from build123d import *

# Parameters (mm, degrees)
SKETCH1_W           = 18.734993996
SKETCH1_H           = 15
BOSS_EXTRUDE1_DEPTH = 26
SKETCH2_R           = 6.5
CUT_EXTRUDE1_DEPTH  = 33.32645975
CHAMFER1_SIZE       = 0.5
SKETCH3_R           = 7
BOSS_EXTRUDE2_DEPTH = 4
SKETCH4_R           = 6
BOSS_EXTRUDE3_DEPTH = 11.5
FILLET1_R           = 1.5


with BuildPart() as part:
    # Sketch1 → Boss-Extrude1 (new body)
    with BuildSketch(Plane.XY):
        Rectangle(SKETCH1_W, SKETCH1_H)
        with BuildLine():
            ThreePointArc((-9.367496998, 7.5), (-12, 0), (-9.367496998, -7.5))
            Line((-9.367496998, -7.5), (-9.367496998, 7.5))
        make_face()
        with BuildLine():
            Line((9.367496998, 7.5), (9.367496998, -7.5))
            ThreePointArc((9.367496998, -7.5), (11.322763885, -3.974294656), (12, 0))
            ThreePointArc((12, 0), (11.322763885, 3.974294656), (9.367496998, 7.5))
        make_face()
    extrude(amount=BOSS_EXTRUDE1_DEPTH)

    # Sketch2 → Cut-Extrude1 (cut, through all)
    with BuildSketch(Plane(origin=(0, 7.5, 0), x_dir=(1, 0, 0), z_dir=(0, 1, 0))):
        with Locations(Location((0, -13, 0), (0, 0, 270))):
            Circle(SKETCH2_R)
    extrude(amount=-CUT_EXTRUDE1_DEPTH, mode=Mode.SUBTRACT)

    # Chamfer1
    chamfer1_edges = [part.edges().sort_by_distance(p)[0] for p in [
        (0, -7.5, 6.5),
        (0, 7.5, 6.5),
    ]]
    chamfer(chamfer1_edges, length=CHAMFER1_SIZE)

    # Sketch3 → Boss-Extrude2 (add)
    with BuildSketch(Plane.XY.offset(26)):
        Circle(SKETCH3_R)
    extrude(amount=BOSS_EXTRUDE2_DEPTH)

    # Sketch4 → Boss-Extrude3 (add)
    with BuildSketch(Plane.XY.offset(30)):
        Circle(SKETCH4_R)
    extrude(amount=BOSS_EXTRUDE3_DEPTH)

    # Fillet1
    # the kernel refuses this fillet: 1.5 mm, written as the material it adds along each edge
    with BuildSketch(Plane(origin=(0, 0, 30), x_dir=(1, 0, 0), z_dir=(0, -1, 0))) as fillet1_piece_1:
        with BuildLine():
            CenterArc((7.5, 1.414213562), FILLET1_R, 180, 70.528779366)
            Line((6, 1.414213562), (6, 0))
            Line((6, 0), (7, 0))
        make_face()
    revolve(axis=Axis((0, 0, 30), (0, 0, 1)))
    # the kernel refuses this fillet: 1.5 mm, written as the material it takes off along each edge
    with BuildSketch(Plane(origin=(0, 0, 41.5), x_dir=(1, 0, 0), z_dir=(0, -1, 0))) as fillet1_2_piece_1:
        with BuildLine():
            CenterArc((6 - FILLET1_R, -FILLET1_R), FILLET1_R, 0, 90)
            Line((6 - FILLET1_R, 0), (6, 0))
            Line((6, 0), (6, -FILLET1_R))
        make_face()
    revolve(axis=Axis((0, 0, 41.5), (0, 0, 1)), mode=Mode.SUBTRACT)

    # Mirror1: read off the stored shape, not the designer's step
    # Mirror1 outline → Mirror1 (revolve)
    with BuildSketch(Plane.XZ):
        with BuildLine():
            ThreePointArc((6, -5.414213562), (6.275255129, -4.548188159), (7, -4))
            Line((7, -4), (7, 0))
            Line((7, 0), (0, 0))
            Line((0, 0), (0, -15.5))
            Line((0, -15.5), (4.5, -15.5))
            ThreePointArc((4.5, -15.5), (5.560660172, -15.060660172), (6, -14))
            Line((6, -14), (6, -5.414213562))
        make_face()
    revolve(axis=Axis((0, 0, 0), (0, 0, 1)))


solid = part.part
Design review of the part built by this model. Coordinates are the model's own, in mm. A direction names the side the tool comes from. Give positions to 0.01 mm unless a question says otherwise; leave off trailing zeros. Write each loop counter-clockwise with the first axis right and the second up, starting at its lowest first coordinate (ties: lowest second). Pieces come first, ordered by that corner, then holes. Notation, with made-up numbers: M -15,7 L -8,7 A23 cw -8,17 Z; hole C -38,2.25 d6. An arc over 180 degrees is marked long. Return JSON: item names as keys, results as strings. Group by question number.
Item 1: The part is to be moulded in two halves that separate along X. For faces 1 (the flat face through (0, 0, 41.5)), 2 (the cylindrical face through (-12, 0, 13)), 3 (the cylindrical face through (1.95, 0.1, 19.2)), 4 (the cylindrical face through (-6, 0, -10)), say which applies: pulls with the +X half, pulls with the -X half, needs draft (parallel to the pull), parting line crosses it, or undercut.
Item 2: Wall thickness on line 1 along Z through (x, y) = (-7.25, 2.5); line 2 along Z through (x, y) = (0.75, -3); line 3 along Z through (x, y) = (1.5, 0.75): over which ranges is each line inside the solid? List them lowest first.
Item 3: Clearance check with flat-ended pins moving along their axes: pin 1 Ø12 at (x, z) = (-4.5, 15.5) entering from +Y; pin 2 Ø1 at (y, z) = (-4, 16.5) entering from +X; pin 3 Ø1 at (x, z) = (-3.5, 32) entering from -Y; pin 4 Ø4 at (y, z) = (0, -4.5) entering from -X. State where each tip first meets the part, or that it passes through.
Item 4: Take a section at C-C (z = -9). Give the boundary of the cut face in (x, y).
Item 5: Take a section at A-A (z = 13). Give the boundary of the cut face in (x, y).
Item 6: Take a section at D-D (x = -8.5). Give the boundary of the cut face in (y, z).
Item 7: Tool access review of faces 5 (the flat face through (-3, -7, 26)), 6 (the flat face through (0, 0, -15.5)), 7 (the cylindrical face through (6.466, -2.681, -1.972)): name each direction out of +Z, -Z, +X, -X, +Y, -Y from which nothing blocks a thin tool from reaching the whole face with its end or side.
Return value:
{
 "1": {"face 1": "needs draft", "face 2": "pulls with the -X half", "face 3": "undercut", "face 4": "parting line crosses it"},
 "2": {"line 1": "z = 0 to 26", "line 2": "z = -15.5 to 6.54, 19.46 to 41.5", "line 3": "z = -15.5 to 6.68, 19.32 to 41.5"},
 "3": {"pin 1": "stops at y = 7.5", "pin 2": "stops at x = 11.48", "pin 3": "stops at y = -5.2", "pin 4": "stops at x = -7"},
 "4": {"outline": "C 0,0 d12"},
 "5": {"outline": "M -9.37,-7.5 L -7,-7.5 L -6.5,-7 L -6.5,7 L -7,7.5 L -9.37,7.5 A12 ccw Z; M 6.5,-7 L 7,-7.5 L 9.37,-7.5 A12 ccw 9.37,7.5 L 7,7.5 L 6.5,7 Z"},
 "6": {"outline": "M -7.5,0 L 7.5,0 L 7.5,26 L -7.5,26 Z"},
 "7": {"face 5": "+Z", "face 6": "-Z, +X, -X, +Y, -Y", "face 7": "-Z"}
}
